Autodesk Inventor part; units mm, degrees
ref_plane "YZ Plane" through (0, 0, 0) normal (1, 0, 0) x (0, 1, 0)
ref_plane "XZ Plane" through (0, 0, 0) normal (0, 1, 0) x (-1, 0, 0)
ref_plane "XY Plane" through (0, 0, 0) normal (0, 0, 1) x (1, 0, 0)
sketch "Sketch1" plane through (0, 0, 0) normal (0, 0, 1) x (1, 0, 0)
  line L0 (-15, 12.5) -> (15, 12.5)
  line L1 (15, 12.5) -> (15, -12.5)
  line L2 (15, -12.5) -> (-15, -12.5)
  line L3 (-15, -12.5) -> (-15, 12.5)
  line L4 (-15, 12.5) -> (15, -12.5) construction
  line L5 (15, 12.5) -> (-15, -12.5) construction
  point P0 (0, 0)
  dimension "d14" = 6
  dimension "d0" = 30
  dimension "d10" = 25
extrude "Extrusion1" add sketch "Sketch1" along normal blind 10
sketch "Sketch2" plane through (0, 0, 10) normal (0, 0, 1) x (1, 0, 0)
  circle A0 centre (0, -1.5) radius 8.1
  line L0 (15, 12.5) -> (-15, 12.5)
  point P0 (0, 12.5)
  dimension "d4" = 16.2
  dimension "d38" = 14
extrude "Extrusion2" cut sketch "Sketch2" against normal blind 5.2
sketch "Sketch3" plane through (0, -1.5, 4.8) normal (0, 0, 1) x (1, 0, 0)
  circle A0 centre (0, 0) radius 4.5
  circle A1 centre (0, 0) radius 8.1
  dimension "d7" = 9
extrude "Extrusion3" cut sketch "Sketch3" against normal blind 5.2 contours A0
sketch "Sketch4" plane through (-15, -12.5, 0) normal (0, -1, 0) x (1, 0, 0)
  line L0 (0, 0) -> (0, 10)
  line L1 (0, 10) -> (30, 10)
  point P0 (15, 0)
  point P1 (4, 5)
  dimension "d11" = 4
  dimension "d12" = 5
hole "Hole1" at (-11, -12.5, 5) direction (0, 1, 0) diameter 4 end through all counterbore diameter 7 counterbore depth 4
sketch "Sketch5" plane through (-15, -12.5, 0) normal (0, -1, 0) x (1, 0, 0)
  line L0 (30, 0) -> (30, 10)
  line L1 (0, 10) -> (30, 10)
  point P0 (15, 0)
  point P1 (26, 5)
  dimension "d20" = 4
  dimension "d21" = 5
hole "Hole2" at (11, -12.5, 5) direction (0, 1, 0) diameter 4 end through all counterbore diameter 7 counterbore depth 4
sketch "Sketch6" plane through (-15, -12.5, 0) normal (0, -1, 0) x (1, 0, 0)
  line L0 (0, 10) -> (30, 10)
  line L1 (30, 0) -> (30, 10)
  point P0 (15, 0)
  point P1 (15, 7.3)
  dimension "d29" = 2.7
  dimension "d30" = 15
hole "Hole3" at (0, -12.5, 7.3) direction (0, 1, 0) diameter 2.7 depth 8 tip angle 118
fillet "Fillet2" radius 0.5 5 edges at (-15, 0, 10) (0, -12.5, 0) (15, -12.5, 5) (-15, -12.5, 5) (0, -12.5, 10)
properties part number "wheel_holder"
Work out the finished part from the listing and answer in its coordinate system (mm). A direction names the side the tool comes from. Round coordinates to 2 decimals unless told otherwise and drop trailing zeros. Loops run counter-clockwise (first coordinate to the right, second up) from the corner with the lowest first, then second, coordinate; pieces in that order, holes last. Notation, with made-up numbers: M 50.5,69 L 55.5,69 A16 cw 55.5,98 Z; hole C 75,41 d3. An arc over 180 degrees is marked long. Use CSV: the item, a comma, the result in double quotes.
Q1. Section D-D, the plane z = 1 is taken. Determine the outline of the cut face in (x, y).
Determined:
outline,"M -15,-12 A0.5 ccw -14.5,-12.5 L 14.5,-12.5 A0.5 ccw 15,-12 L 15,12.5 L -15,12.5 Z; hole C 0,-1.5 d9"
Q2. Section C-C, the plane y = 10.5 is taken. Determine the outline of the cut face in (x, z).
Determined:
outline,"M -15,0 L 15,0 L 15,10 L -14.5,10 A0.5 ccw -15,9.5 Z; hole C -11,5 d4; hole C 11,5 d4"
Q3. Consider L1, parallel to Z at x = -11, y = -9.65; L2, parallel to Y at x = 0, z = 2.25; L3, parallel to X at y = -3.5, z = 3.5. Determine where each line is inside the solid, lowest interval first.
Determined:
L1,"0 to 1.5, 8.5 to 10"
L2,"-12.5 to -6, 3 to 12.5"
L3,"-15 to -12.32, -9.68 to -4.03, 4.03 to 9.68, 12.32 to 15"
Q4. A tool of negligible diameter and unlimited length cuts with its end or side. For faces 1 (the cylindrical face through (-1.756, -9.407, 7.436)), 2 (the cylindrical face through (9, 2, 5)), 3 (the cylindrical face through (-0.406, -10.972, 6.012)), from which of +Z, -Z, +X, -X, +Y, -Y can it reach the whole face along a straight path? Write none if from no direction.
Determined:
face 1,"+Z"
face 2,"+Y, -Y"
face 3,"-Y"
Q5. Section B-B, the plane x = 11 is taken. Determine the outline of the cut face in (y, z).
Determined:
outline,"M -12.5,0.5 A0.5 ccw -12,0 L 12.5,0 L 12.5,3 L -8.5,3 L -8.5,1.5 L -12.5,1.5 Z; M -12.5,8.5 L -8.5,8.5 L -8.5,7 L 12.5,7 L 12.5,10 L -12,10 A0.5 ccw -12.5,9.5 Z"
Q6. Each of these flat-tipped pins is pushed along its axis until it touches: pin 1 (8 mm diameter, centred on x = 0, y = -1.5, fed in from +Z); pin 2 (2 mm diameter, centred on x = -9.5, z = 4.5, fed in from -Y). Where does it stop, or does it pass through?
Determined:
pin 1,"through"
pin 2,"y = -8.5"
Q7. Section A-A, the plane y = -1.5 is taken. Determine the outline of the cut face in (x, z).
Determined:
outline,"M -15,0 L -4.5,0 L -4.5,4.8 L -8.1,4.8 L -8.1,10 L -14.5,10 A0.5 ccw -15,9.5 Z; M 4.5,0 L 15,0 L 15,10 L 8.1,10 L 8.1,4.8 L 4.5,4.8 Z; hole C -11,5 d4; hole C 11,5 d4"
Q8. The mould has two halves that part along Z. Classify faces 4 (the cylindrical face through (-7.583, -10.472, 5.759)), 5 (the cylindrical face through (-0.59, 2.96, 2.43)), 6 (the flat face through (-4, 3, 0)): pulls with the +Z half, pulls with the -Z half, needs draft (parallel to the pull), parting line crosses it, or undercut.
Determined:
face 4,"undercut"
face 5,"needs draft"
face 6,"pulls with the -Z half"
